Design review of the part built by this model. Coordinates are the model's own, in mm. A direction names the side the tool comes from. Round coordinates to 2 decimals unless told otherwise and drop trailing zeros. Order: outer loops, then holes, each group sorted by start corner. A loop starts at its lowest first (then second) coordinate and runs counter-clockwise, first axis right, second up. Notation, with made-up numbers: M 77,87.25 L 93,87.25 A14 cw 93,106.25 Z; hole C -12.75,45.5 d6. An arc over 180 degrees is marked long. Write item = value, one per line. Start each with the question number.
Autodesk Inventor part; units mm, degrees
ref_plane "YZ Plane" through (0, 0, 0) normal (1, 0, 0) x (0, 1, 0)
ref_plane "XZ Plane" through (0, 0, 0) normal (0, 1, 0) x (-1, 0, 0)
ref_plane "XY Plane" through (0, 0, 0) normal (0, 0, 1) x (1, 0, 0)
sketch "Sketch1" plane through (0, 0, 0) normal (0, 0, 1) x (1, 0, 0)
  circle A0 centre (12.5, 11.5) radius 1.6
  line L0 (0, 0) -> (18, 0)
  line L1 (0, 0) -> (0, 3)
  arc A1 (18, 11.5) -> (7.7369, 14.25) centre (12.5, 11.5) ccw
  line L2 (12.5, 11.5) -> (7.7369, 14.25) construction
  line L3 (12.5, 11.5) -> (18, 11.5) construction
  line L4 (7.7369, 14.25) -> (0, 3)
  line L5 (18, 11.5) -> (18, 0)
  dimension "d17" = 3
  dimension "d19" = 11.5
  dimension "d23" = 90
  dimension "d25" = 12.5
  dimension "d31" = 5.5
  dimension "d32" = 150
  dimension "d49" = 3.2
  dimension "d51" = 18
extrude "Extrusion1" add sketch "Sketch1" along normal blind 4.5
sketch "Sketch4" plane through (0, 0, 4.5) normal (0, 0, 1) x (1, 0, 0)
  line L0 (0, 3) -> (0, 0)
  line L1 (18, 0) -> (18, 3)
  line L2 (0, 0) -> (18, 0)
  line L3 (18, 0) -> (18, 3)
  line L4 (18, 3) -> (0, 3)
  line L5 (0, 3) -> (0, 0)
  line L6 (18, 0) -> (18, 11.5)
extrude "Extrusion2" add sketch "Sketch4" along normal blind 4.5
sketch "Sketch5" plane through (0, 0, 0) normal (0, -1, 0) x (1, 0, 0)
  circle A0 centre (5, 4.8) radius 1.6
  circle A1 centre (13, 4.8) radius 1.6
  line L0 (0, 0) -> (18, 0)
  line L1 (0, 4.5) -> (0, 9)
  point P0 (20.0001, 0)
  dimension "d13" = 3.2
  dimension "d14" = 3.2
  dimension "d38" = 4.8
  dimension "d39" = 4.8
  dimension "d50" = 8
  dimension "d52" = 5
extrude "Extrusion3" cut sketch "Sketch5" against normal through all
sketch "Sketch6" plane through (0, 3, 9) normal (0, 1, 0) x (1, 0, 0)
  circle A0 centre (5, 4.2) radius 1.6
  circle A1 centre (5, 4.2) radius 3
  circle A2 centre (13, 4.2) radius 1.6
  circle A3 centre (13, 4.2) radius 3
  line L0 (0, 9) -> (18, 9)
  point P0 (20.0001, 9)
  dimension "d34" = 6
  dimension "d35" = 6
  dimension "d40" = 4.8
  dimension "d41" = 4.8
extrude "Extrusion4" cut sketch "Sketch6" along normal up to next
sketch "Sketch7" plane through (0, 0, 0) normal (0, -1, 0) x (1, 0, 0)
  line L0 (0, 0) -> (0, 9)
  line L1 (2.042, 0) -> (0, 0)
  line L2 (0, 0) -> (0, 9)
  line L3 (0, 9) -> (2.042, 9)
  line L4 (2.042, 9) -> (2.042, 0)
extrude "Extrusion5" cut sketch "Sketch7" against normal up to next
properties part number "lower_deck_shaft_mount_v4_printing"
(1) For faces 1 (the face through (5.98, 7.445, 1.965)), 2 (the face through (4.93, 10.17, 1.16)), 3 (the face through (9, 10, 4.5)), list the 3-axis set-ups (+Z, -Z, +X, -X, +Y, -Y) from which the entire face can be reached by the end or side of a thin tool; tool diameter is ignored.
(2) Draft analysis for pull direction X (two halves, no side actions). For faces 4 (the face through (10, 7, 0)), 5 (the face through (13.9, 9.9, 1.94)), 6 (the face through (2.042, 2, 4)), state which applies: pulls with the +X half, pulls with the -X half, needs draft (parallel to the pull), parting line crosses it, or undercut.
(3) For line 1 along Y through (x, z) = (12.5, 1.75); line 2 along Z through (x, y) = (13, 2); line 3 along Z through (x, y) = (8.5, 13.5), list the stretches that pass through material, from the lowest coordinate up. Write a range as [from, to].
(4) Consider section A-A, the plane z = 4.8. Write out the cut boundary in (x, y), then the cut area to 3 significant figures.
(5) Insertion check: pin 1 (6 mm diameter, centred on x = 6, y = 13.5, fed in from +Z); pin 2 (4 mm diameter, centred on x = 12.5, y = 11.5, fed in from +Z); pin 3 (1.5 mm diameter, centred on x = 6, z = 4.5, fed in from +Y). Each pin has a flat end and moves straight along its axis. Give the tip position at first contact, or say it passes through.
(6) Consider section D-D, the plane x = 5. Write out the cut boundary in (y, z).
(7) Consider section C-C, the plane y = 11. Write out the cut boundary in (x, z), then the cut area to 3 significant figures.
(8) Consider section B-B, the plane x = 12.5. Write out the cut boundary in (y, z).
Completed:
q1.face_1 = +Z, +Y
q1.face_2 = +Z, -Z, -X, +Y
q1.face_3 = +Z, +X, -X, +Y
q2.face_4 = needs draft
q2.face_5 = undercut
q2.face_6 = pulls with the -X half
q3.line_1 = [0, 9.9], [13.1, 17]
q3.line_2 = [0, 3.2], [6.4, 9]
q3.line_3 = [0, 4.5]
q4.outline = M 2.04,0 L 3.4,0 L 3.4,3 L 2.04,3 Z; M 6.6,0 L 11.4,0 L 11.4,3 L 6.6,3 Z; M 14.6,0 L 18,0 L 18,3 L 14.6,3 Z
q4.area = 28.7 mm2
q5.pin_1 = 4.5
q5.pin_2 = 3.14
q5.pin_3 = 3
q6.outline = M 0,0 L 10.27,0 L 10.27,1.8 L 3,1.8 L 3,3.2 L 0,3.2 Z; M 0,6.4 L 3,6.4 L 3,9 L 0,9 Z
q7.outline = M 5.5,0 L 10.98,0 L 10.98,2.58 A3 cw 10.02,4.5 L 7.98,4.5 A3 cw 5.5,1.84 Z; M 14.02,0 L 18,0 L 18,4.5 L 15.98,4.5 A3 cw 14.02,1.98 Z
q7.area = 33.1 mm2
q8.outline = M 0,0 L 9.9,0 L 9.9,1.84 L 3,1.84 L 3,3.28 L 0,3.28 Z; M 0,6.32 L 3,6.32 L 3,9 L 0,9 Z; M 13.1,0 L 17,0 L 17,1.84 L 13.1,1.84 Z
